```python
from build123d import *

# Parameters (mm, degrees)
F0_W           = 30
F0_H           = 500
F1_DEPTH       = 30
F2_D           = 10
F2_CSINK_D     = 12
F2_CSINK_ANGLE = 90


with BuildPart() as f1:
    # F0 (on Front) → F1 (new body)
    with BuildSketch(Plane.XZ):
        with Locations((0.3963927738, 157.8636374871)):
            Rectangle(F0_W, F0_H)
    extrude(amount=F1_DEPTH)

    # F2 (through all)
    with Locations(Plane(origin=(0, 0, 0), x_dir=(1, 0, 0), z_dir=(0, 1, 0))):
        with Locations((0, -362.025141716)):
            CounterSinkHole(F2_D / 2, F2_CSINK_D / 2, counter_sink_angle=F2_CSINK_ANGLE)


solid = f1.part
```
Verification items for the finished model (mm, model axes). Give positions to 0.01 mm unless a question says otherwise; leave off trailing zeros. Loops run counter-clockwise (first coordinate to the right, second up) from the corner with the lowest first, then second, coordinate; pieces in that order, holes last.
1. Section check A-A, the plane x = 0. Enter the section's corners in (y, z), then the cut area to 3 significant figures.
2. Go/stop test with flat-tipped pins: pin 1 Ø11.5 at (x, z) = (0, 362.03) entering from +Y; pin 2 Ø1.5 at (x, z) = (12, 27.5) entering from +Y. Record where each tip stops, or that it passes through.
3. Mould release check, pull along Z, two halves, no side actions. Record for faces 1 (the flat face through (0, -15, -92.136)), 2 (the cylindrical face through (-2.69, -15.7, 357.81)), 3 (the flat face through (0, -15, 407.864)), 4 (the flat face through (15.396, -15, 154)): released by +Z, released by -Z, zero draft, split by the parting line, or undercut.
4. Thickness scan on line 1 (Z direction, x = 0, y = -12.5); line 2 (Z direction, x = -2.25, y = -24.5). Record the ranges inside material, lowest first.
Geometry says:
1. outline: (-30, -92.14) - (0, -92.14) - (0, 356.03) - (-1, 357.03) - (-30, 357.03) - close; (-30, 367.03) - (-1, 367.03) - (0, 368.03) - (0, 407.86) - (-30, 407.86) - close
1. area: 14,700 mm2
2. pin 1: stops at y = -0.25
2. pin 2: stops at y = 0
3. face 1: released by -Z
3. face 2: undercut
3. face 3: released by +Z
3. face 4: zero draft
4. line 1: z = -92.14 to 357.03, 367.03 to 407.86
4. line 2: z = -92.14 to 357.56, 366.49 to 407.86
